Check sheet for the modelled part. Datum: model origin and axes. Units: mm. A direction names the side the tool comes from. Coordinates: 2 decimals unless noted, no trailing zeros. Write each loop counter-clockwise with the first axis right and the second up, starting at its lowest first coordinate (ties: lowest second). Pieces come first, ordered by that corner, then holes. Notation, with made-up numbers: M 18.5,-11 L 59.5,-11 A17 ccw 59.5,11 Z; hole C -17,-11.75 d4. An arc over 180 degrees is marked long. Answer as CSV lines item,"result". Start each with the question number.
Q1. Depth check by flat-ended pin: pin 1 Ø10 at (y, z) = (7.5, 42) entering from +X; pin 2 Ø11.5 at (x, y) = (26.5, 4) entering from -Z. Enter the tip coordinate at first touch or a pass-through.
Q2. Thickness scan on line 1 along Z through (x, y) = (6.5, -8); line 2 along Y through (x, z) = (0, 47) (3 decimals); line 3 along X through (y, z) = (0.5, 5). Record the ranges inside material, lowest first. Write a range as from..to.
Q3. Sectioned sample at D-D, the plane y = 11.5. Record the cut outline in (x, z), then the cut area to 3 significant figures.
Q4. Sectioned sample at B-B, the plane z = 29.5. Record the cut outline in (x, y) (3 decimals), then the cut area to 3 significant figures.
Q5. Sectioned sample at A-A, the plane y = 0. Record the cut outline in (x, z) (3 decimals).
Q6. Sectioned sample at C-C, the plane x = -7.5. Record the cut outline in (y, z), then the cut area to 3 significant figures.
Q7. Mould release check, pull along Z, two halves, no side actions. Record for faces 5 (the cylindrical face through (-7.559, -5.796, 47.669)), 6 (the flat face through (5, 9, 38.1)), 7 (the flat face through (5, 9, 44.45)), 8 (the flat face through (27, 0, 19.05)): pulls with the +Z half, pulls with the -Z half, needs draft (parallel to the pull), parting line crosses it, or undercut.
Q8. Access from +Z, -Z, +X, -X, +Y, -Y to the whole of each face (thin tool, end or side, straight path). Record for faces 1 (the flat face through (27, 0, 31.75)), 2 (the cylindrical face through (-15.12, -11.59, 41.14)), 3 (the cylindrical face through (-2.75, -12.4, 41.32)), 4 (the cylindrical face through (-15.12, -11.59, 9.39)).
from build123d import *

# Parameters (mm, degrees)
F0_R      = 19.05
F1_DEPTH  = 19.05
F3_DEPTH  = 12.7
F4_R      = 19.05
F5_DEPTH  = 6.35
F6_R      = 9.525
F7_DEPTH  = 57.15
F8_R      = 19.05
F9_DEPTH  = 6.35
F10_R     = 12.7
F11_DEPTH = 6.35
F12_R     = 19.05
F13_DEPTH = 6.35
F14_R     = 9.525
F15_DEPTH = 6.35


with BuildPart() as f1:
    # F0 (on Top) → F1 (new body)
    with BuildSketch(Plane.XY):
        Circle(F0_R)
    extrude(amount=F1_DEPTH)

    # F2 (on face) → F3 (join)
    with BuildSketch(Plane.XY.offset(19.05)):
        Polygon((38.1, 19.05), (0, 19.05), (-38.1, 19.05), (-38.1, -19.05), (0, -19.05), (38.1, -19.05), align=None)
    extrude(amount=F3_DEPTH)

    # F4 (on face) → F5 (join)
    with BuildSketch(Plane.XY.offset(31.75)):
        Circle(F4_R)
    extrude(amount=F5_DEPTH)

    # F6 (on face) → F7 (cut)
    with BuildSketch(Plane.XY.offset(38.1)):
        Circle(F6_R)
    extrude(amount=-F7_DEPTH, mode=Mode.SUBTRACT)

    # F8 (on face) → F9 (join)
    with BuildSketch(Plane.XY.offset(38.1)):
        Circle(F8_R)
    extrude(amount=F9_DEPTH)

    # F10 (on face) → F11 (cut)
    with BuildSketch(Plane.XY.offset(44.45)):
        Circle(F10_R)
    extrude(amount=-F11_DEPTH, mode=Mode.SUBTRACT)

    # F12 (on face) → F13 (join)
    with BuildSketch(Plane.XY.offset(44.45)):
        Circle(F12_R)
    extrude(amount=F13_DEPTH)

    # F14 (on face) → F15 (cut)
    with BuildSketch(Plane.XY.offset(50.8)):
        Circle(F14_R)
    extrude(amount=-F15_DEPTH, mode=Mode.SUBTRACT)


solid = f1.part
Output:
1,pin 1,"stops at x = 18.89"
1,pin 2,"stops at z = 19.05"
2,line 1,"z = 0..38.1, 44.45..50.8"
2,line 2,"y = -19.05..-9.525, 9.525..19.05"
2,line 3,"x = -19.04..-9.51, 9.51..19.04"
3,outline,"M -38.1,19.05 L -15.19,19.05 L -15.19,0 L 15.19,0 L 15.19,19.05 L 38.1,19.05 L 38.1,31.75 L 15.19,31.75 L 15.19,50.8 L -15.19,50.8 L -15.19,31.75 L -38.1,31.75 Z; hole M -5.39,38.1 L 5.39,38.1 L 5.39,44.45 L -5.39,44.45 Z"
3,area,"2,060 mm^2"
4,outline,"M -38.1,-19.05 L 38.1,-19.05 L 38.1,19.05 L -38.1,19.05 Z; hole C 0,0 d19.05"
4,area,"2,620 mm^2"
5,outline,"M -38.1,19.05 L -19.05,19.05 L -19.05,0 L -9.525,0 L -9.525,38.1 L -12.7,38.1 L -12.7,44.45 L -9.525,44.45 L -9.525,50.8 L -19.05,50.8 L -19.05,31.75 L -38.1,31.75 Z; M 9.525,0 L 19.05,0 L 19.05,19.05 L 38.1,19.05 L 38.1,31.75 L 19.05,31.75 L 19.05,50.8 L 9.525,50.8 L 9.525,44.45 L 12.7,44.45 L 12.7,38.1 L 9.525,38.1 Z"
6,outline,"M -19.05,19.05 L -17.51,19.05 L -17.51,0 L -5.87,0 L -5.87,38.1 L -10.25,38.1 L -10.25,44.45 L -5.87,44.45 L -5.87,50.8 L -17.51,50.8 L -17.51,31.75 L -19.05,31.75 Z; M 5.87,0 L 17.51,0 L 17.51,19.05 L 19.05,19.05 L 19.05,31.75 L 17.51,31.75 L 17.51,50.8 L 5.87,50.8 L 5.87,44.45 L 10.25,44.45 L 10.25,38.1 L 5.87,38.1 Z"
6,area,"1,170 mm^2"
7,face 5,"needs draft"
7,face 6,"undercut"
7,face 7,"undercut"
7,face 8,"pulls with the -Z half"
8,face 1,"+Z, +X"
8,face 2,"+Z"
8,face 3,"none"
8,face 4,"-Z"
